```python
from build123d import *

# Parameters (mm, degrees)
RECESS_CUT_EXTRUDE1_DEPTH = 2.42
SKETCH7_R                 = 2.8
RECESS_CUT_EXTRUDE2_DEPTH = 0.363


with BuildPart() as part:
    # Sketch1 → BODY (revolve)
    with BuildSketch(Plane.XY, mode=Mode.PRIVATE) as body_sk:
        Polygon((0, 0), (3.4, 0), (3.4, 60), (6, 60), (6, 64.6), (0, 64.6), align=None)
    revolve(body_sk.sketch.rotate(Axis((0, 0, 0), (0, 1, 0)), 90), axis=Axis((0, 0, 0), (0, 1, 0)))

    # Sketch2 → HEAD-CUT (revolve, cut)
    with BuildSketch(Plane.XY, mode=Mode.PRIVATE) as head_cut_sk:
        with BuildLine():
            ThreePointArc((10, 55.45), (7.071067812, 62.521067812), (0, 65.45))
            Line((0, 65.45), (0, 65.93216157))
            Line((0, 65.93216157), (10, 65.93216157))
            Line((10, 65.93216157), (10, 55.45))
        make_face()
    revolve(head_cut_sk.sketch.rotate(Axis((0, 0, 0), (0, 1, 0)), 90), axis=Axis((0, 0, 0), (0, 1, 0)), mode=Mode.SUBTRACT)

    # Sketch4 → GAP (revolve, cut)
    with BuildSketch(Plane.XY, mode=Mode.PRIVATE) as gap_sk:
        with BuildLine():
            Line((-3.4, 58), (-3.251503787, 59.75))
            ThreePointArc((-3.251503787, 59.75), (-3.28566705, 59.89880979), (-3.4, 60))
            Line((-3.4, 60), (-3.4, 58))
        make_face()
    revolve(gap_sk.sketch.rotate(Axis((0, 0, 0), (0, 1, 0)), 270), axis=Axis((0, 0, 0), (0, 1, 0)), mode=Mode.SUBTRACT)

    # Sketch5 → Recess-Cut-Extrude1 (cut)
    with BuildSketch(Plane(origin=(0, 64.6, 0), x_dir=(-1, 0, 0), z_dir=(0, 1, 0))):
        with BuildLine():
            add(Edge.make_bspline(
                [(2.8, 0), (2.645109866, -0.023911085), (1.670994331, 0.199786237), (1.414118172, -1.106473263), (-0.315407204, -3.117616193), (-0.08378741, -0.750252113), (-1.3658447, -0.443842911), (-2.797125263, -0.196308398), (-2.80002409, 0.001077292), (-2.800023768, 0.001616003)],
                knots=[0.179018134, 0.179018134, 0.179018134, 0.179018134, 0.237467971, 0.292040128, 0.415648105, 0.507114761, 0.541693416, 0.662364746, 0.662694958, 0.662694958, 0.662694958, 0.662694958], degree=3))
            ThreePointArc((2.8, 0), (2.799094521, 0.071202971), (2.796378669, 0.142359889))
            add(Edge.make_bspline(
                [(1.4, 2.424871131), (1.513938157, 2.323513219), (1.329282824, 1.267778391), (2.57149917, 0.398112713), (2.796378669, 0.142359889)],
                knots=[0, 0, 0, 0, 0.052176783, 0.148749777, 0.148749777, 0.148749777, 0.148749777], degree=3))
            ThreePointArc((1.4, 2.424871131), (1.379598676, 2.436535962), (1.359100168, 2.448029153))
            add(Edge.make_bspline(
                [(-2.800023768, 0.001616003), (-2.799909028, 0.193193204), (-0.88460249, 0.55646964), (-0.772921937, 2.873205542), (0.205731927, 1.792311947), (1.119461988, 2.526850423), (1.359100168, 2.448029153)],
                knots=[0.662694958, 0.662694958, 0.662694958, 0.662694958, 0.780125533, 0.878673095, 0.910848295, 0.994606061, 0.994606061, 0.994606061, 0.994606061], degree=3))
        make_face()
    extrude(amount=-RECESS_CUT_EXTRUDE1_DEPTH, mode=Mode.SUBTRACT)

    # Sketch3 → DRILL-CUT (revolve, cut)
    with BuildSketch(Plane.XY):
        Polygon((0, 60.936476343), (2.153846154, 62.18), (0, 62.18), align=None)
    revolve(axis=Axis((0, 0, 0), (0, 1, 0)), mode=Mode.SUBTRACT)

    # Sketch7 → Recess-Cut-Extrude2 (cut)
    with BuildSketch(Plane(origin=(0, 64.6, 0), x_dir=(-1, 0, 0), z_dir=(0, 1, 0))):
        with Locations(Location((0, 0, 0), (0, 0, 90))):
            Circle(SKETCH7_R)
    extrude(amount=-RECESS_CUT_EXTRUDE2_DEPTH, mode=Mode.SUBTRACT)


solid = part.part
```
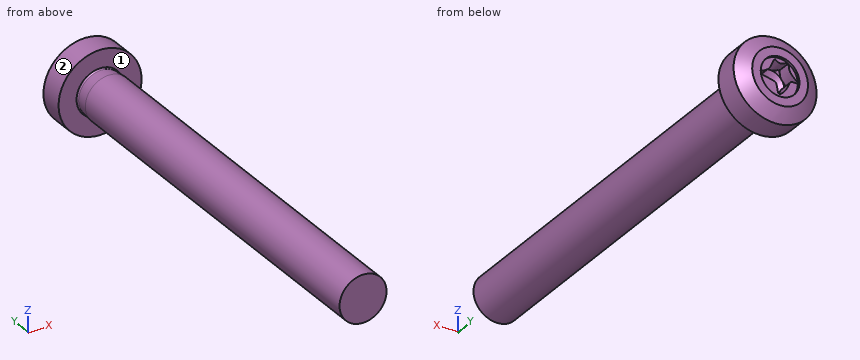
Verification items for the finished model (mm, model axes). Face numbers are marked on the shaded views. A direction names the side the tool comes from. Round coordinates to 2 decimals unless told otherwise and drop trailing zeros. Order: outer loops, then holes, each group sorted by start corner. A loop starts at its lowest first (then second) coordinate and runs counter-clockwise, first axis right, second up.
1) Material ranges on line 1 (Y direction, x = 3.5, z = -2); line 2 (X direction, y = 44.5, z = -1.75); line 3 (X direction, y = 7, z = -3), recorded low to high.
Geometry says:
line 1: y = 60 to 64.6
line 2: x = -2.92 to 2.92
line 3: x = -1.6 to 1.6
2) Cross-section at B-B, the plane z = 4.75. Record the cut outline in (x, y).
Geometry says:
outline: (-3.67, 60) - (3.67, 60) - (3.67, 63.45) arc R8.8 ccw to (-3.67, 63.45) - close
3) Cross-section at A-A, the plane y = 46. Record the cut outline in (x, z).
Geometry says:
outline: circle Ø6.8 at (0, 0)
4) Tool access check on the marked faces 1 and 2. Record the directions out of +Z, -Z, +X, -X, +Y, -Y that give a thin tool (end or side, any length) a straight path to the whole face; none if there is none.
Geometry says:
face 1: -Y
face 2: +Y, -Y
5) Cross-section at C-C, the plane x = 4.75. Record the cut outline in (y, z), plus the area to 3 significant figures.
Geometry says:
outline: (60, -3.67) - (63.45, -3.67) arc R8.8 ccw to (63.45, 3.67) - (60, 3.67) - close
area: 29.2 mm2
6) Depth check by flat-ended pin: pin 1 (0.5 mm diameter, centred on x = -1, z = 2, fed in from +Y); pin 2 (1.5 mm diameter, centred on y = 30.5, z = 1, fed in from +X); pin 3 (1.5 mm diameter, centred on y = 13.5, z = -1, fed in from -X). Enter the tip coordinate at first touch or a pass-through.
Geometry says:
pin 1: stops at y = 62.18
pin 2: stops at x = 3.39
pin 3: stops at x = -3.39
